Part print with two shaded views. Sizes in mm from the minimum x, y, z corner. A direction names the side the tool comes from. Round coordinates to 2 decimals unless told otherwise and drop trailing zeros. Write each loop counter-clockwise with the first axis right and the second up, starting at its lowest first coordinate (ties: lowest second). Pieces come first, ordered by that corner, then holes. Notation, with made-up numbers: (84.5, 29) - (118.5, 29) arc R34 cw to (118.5, 66) - close; hole circle Ø10 at (20, -19). An arc over 180 degrees is marked (long way). Answer as a JSON object with one key per item and string values. Group by question number.
Item 1: Flat gauge pins, fed straight in: pin 1 (3 mm diameter, centred on x = 73, y = 20.5, fed in from +Z); pin 2 (15 mm diameter, centred on x = 65, y = 19, fed in from -Z); pin 3 (7.5 mm diameter, centred on x = 97, y = 20.5, fed in from +Z); pin 4 (1.5 mm diameter, centred on y = 17, z = 48.5, fed in from -X). Where does each tip first touch, or does it go through?
Item 2: Probe line 1 (X direction, y = 15.5, z = 54); line 2 (X direction, y = 14, z = 5); line 3 (Y direction, x = 79.25, z = 45). List the from-to ranges inside material, lowest first. Write a range as from..to.
Item 3: Slice it at C-C, the plane y = 15. List the corners of the cut face in (x, z), then the cut area to 3 significant figures.
Item 4: Slice it at A-A, the plane z = 8. List the corners of the cut face in (x, y), then the cut area to 3 significant figures.
Item 5: Slice it at B-B, the plane x = 76.5. List the corners of the cut face in (y, z) (1 decimal), then the cut area to 3 significant figures.
Item 6: Two-plate mould, pull along Y, no slides. Class the marked faces 1, 2 and 3: +Y half, -Y half, draft (parallel to the pull), parting line (faces both ways), or undercut.
Item 7: Which spindle directions (+Z, -Z, +X, -X, +Y, -Y) get a long thin tool onto all of the face, cutting with end or side? Do the marked faces 4, 5, 6 and 7. Say none if no direction does.
Item 8: Slice it at D-D, the plane z = 45. List the corners of the cut face in (x, y).
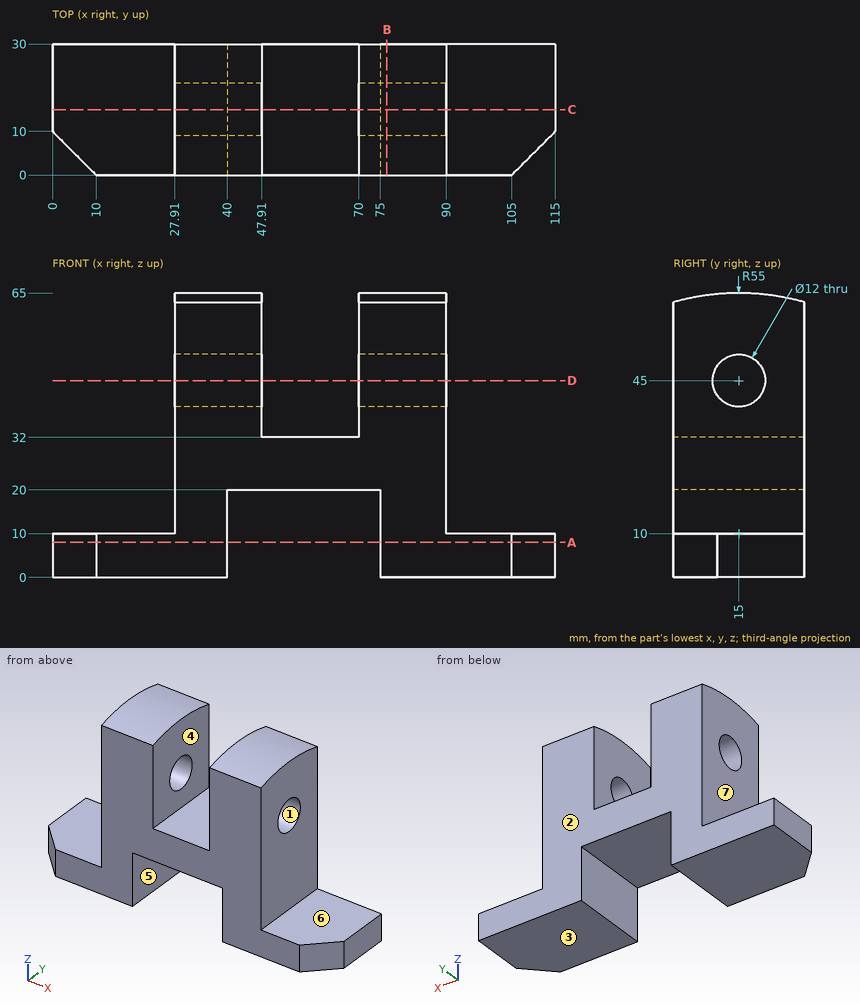
Geometry says:
{
 "1": {"pin 1": "stops at z = 64.85", "pin 2": "stops at z = 20", "pin 3": "stops at z = 10", "pin 4": "passes through"},
 "2": {"line 1": "x = 27.91..47.91, 70..90", "line 2": "x = 0..40, 75..115", "line 3": "y = 0..9, 21..30"},
 "3": {"outline": "(0, 0) - (40, 0) - (40, 20) - (75, 20) - (75, 0) - (115, 0) - (115, 10) - (90, 10) - (90, 39) - (70, 39) - (70, 32) - (47.91, 32) - (47.91, 39) - (27.91, 39) - (27.91, 10) - (0, 10) - close; (27.91, 51) - (47.91, 51) - (47.91, 65) - (27.91, 65) - close; (70, 51) - (90, 51) - (90, 65) - (70, 65) - close", "area": "2,660 mm^2"},
 "4": {"outline": "(0, 10) - (10, 0) - (40, 0) - (40, 30) - (0, 30) - close; (75, 0) - (105, 0) - (115, 10) - (115, 30) - (75, 30) - close", "area": "2,300 mm^2"},
 "5": {"outline": "(0, 0) - (30, 0) - (30, 62.9) arc R55 ccw to (0, 62.9) - close; hole circle Ø12 at (15, 45)", "area": "1,820 mm^2"},
 "6": {"face 1": "undercut", "face 2": "+Y half", "face 3": "draft"},
 "7": {"face 4": "+Z, +Y, -Y", "face 5": "-Z, +Y, -Y", "face 6": "+Z, +X, +Y, -Y", "face 7": "+Z, -X, +Y, -Y"},
 "8": {"outline": "(27.91, 0) - (47.91, 0) - (47.91, 9) - (27.91, 9) - close; (27.91, 21) - (47.91, 21) - (47.91, 30) - (27.91, 30) - close; (70, 0) - (90, 0) - (90, 9) - (70, 9) - close; (70, 21) - (90, 21) - (90, 30) - (70, 30) - close"}
}
